Autodesk Inventor part; units mm, degrees
ref_plane "YZ Plane" through (0, 0, 0) normal (1, 0, 0) x (0, 1, 0)
ref_plane "XZ Plane" through (0, 0, 0) normal (0, 1, 0) x (-1, 0, 0)
ref_plane "XY Plane" through (0, 0, 0) normal (0, 0, 1) x (1, 0, 0)
sketch "Sketch1" plane through (0, 0, 0) normal (0, 1, 0) x (-1, 0, 0)
  line L0 (0, 0) -> (180, 0)
  line L1 (180, 0) -> (180, -180)
  line L2 (180, -180) -> (0, -180)
  line L3 (0, -180) -> (0, 0)
  dimension "d0" = 180
  dimension "d1" = 180
extrude "Extrusion1" add sketch "Sketch1" along normal blind 5
sketch "Sketch2" plane through (0, 5, 0) normal (0, 1, 0) x (1, 0, 0)
  line L0 (-165, 165) -> (-15, 165)
  line L1 (-15, 165) -> (-15, 15)
  line L2 (-15, 15) -> (-165, 15)
  line L3 (-165, 15) -> (-165, 165)
  line L4 (-180, 180) -> (-180, 0)
  point P0 (0, 0)
  dimension "d4" = 150
  dimension "d5" = 150
  dimension "d6" = 15
  dimension "d7" = 15
extrude "Extrusion2" cut sketch "Sketch2" against normal blind 2
chamfer "Chamfer1" distance 2 angle 45 4 edges at (-180, 2.5, 0) (-180, 2.5, -180) (0, 2.5, -180) (0, 2.5, 0)
properties part number "MouldBase20"
Could you check a few things on this model? Use its own coordinates, in mm. Coordinates: 2 decimals unless noted, no trailing zeros. Loops run counter-clockwise (first coordinate to the right, second up) from the corner with the lowest first, then second, coordinate; pieces in that order, holes last.
1. For P1, Ø1.5, axis at x = -161, z = -32.5, coming from the +Y side, with a flat end and sliding along its axis, tell me the tip position at first contact or that it passes through.
2. Imagine slicing it at C-C (x = -103.5). Please give me the cut outline in (y, z).
3. We'd pull the mould along Z, two halves only. Please class faces 1 (the face through (0, 2, -91)), 2 (the face through (-91, 3, -91)), 3 (the face through (-91, 2, -180)): released by +Z, released by -Z, zero draft, split by the parting line, or undercut.
4. I need wall thicknesses on L1, parallel to Z at x = -51, y = 3.35; L2, parallel to Y at x = -27, z = -49. Which ranges of each line are inside material? Lowest first, please.
5. Imagine slicing it at B-B (z = -26). Please give me the cut outline in (x, y).
6. Imagine slicing it at A-A (y = 4.15). Please give me the cut outline in (x, z).
Computed values:
1. P1: stops at y = 3
2. outline: (0, -180) - (5, -180) - (5, -165) - (3, -165) - (3, -15) - (5, -15) - (5, 0) - (0, 0) - close
3. face 1: zero draft
3. face 2: undercut
3. face 3: released by -Z
4. L1: z = -180 to -165, -15 to 0
4. L2: y = 0 to 3
5. outline: (-180, 0) - (0, 0) - (0, 5) - (-15, 5) - (-15, 3) - (-165, 3) - (-165, 5) - (-180, 5) - close
6. outline: (-180, -178) - (-178, -180) - (-2, -180) - (0, -178) - (0, -2) - (-2, 0) - (-178, 0) - (-180, -2) - close; hole (-165, -165) - (-15, -165) - (-15, -15) - (-165, -15) - close
